Geometry check sheet. Reference: the model listing, model coordinates, mm. A direction names the side the tool comes from. Round coordinates to 2 decimals unless told otherwise and drop trailing zeros. Order: outer loops, then holes, each group sorted by start corner. A loop starts at its lowest first (then second) coordinate and runs counter-clockwise, first axis right, second up.
(1) Cross-section at B-B on z = 23. Enter the section's corners in (x, y).
(2) Cross-section at A-A on x = 0. Enter the section's corners in (y, z), and give its area (3 significant figures).
(3) Draft check along Y on faces 4 (the face through (-17.62, 0.55, 74.7)), 5 (the face through (-0.521, -35.716, 12.325)), 6 (the face through (17.55, 43.02, 36.1)), 7 (the face through (0, -44.45, 35)). Enter one of: pulls with the +Y half, pulls with the -Y half, needs draft (parallel to the pull), parting line crosses it, or undercut.
(4) Thickness scan on L1, parallel to Y at x = 0, z = 9; L2, parallel to X at y = -31.75, z = 5; L3, parallel to Z at x = -0.5, y = 19.05. Record the ranges inside material, lowest first.
(5) Set-up check for faces 1 (the face through (-5.95, 19, 51)), 2 (the face through (0, 44.45, 35)), 3 (the face through (-0.521, 27.784, 12.325)): record each of +Z, -Z, +X, -X, +Y, -Y from which the full face is reachable in a straight line by a thin tool's end or side.
(6) Cross-section at C-C on z = 50.8. Enter the section's corners in (x, y), and give its area (3 significant figures).
(7) Gauge pin test, flat ends, axial feed: P1, Ø9, axis at x = 0, y = 31.75, coming from the -Z side; P2, Ø4, axis at x = 1, y = 30.5, coming from the -Z side; P3, Ø2.5, axis at y = -18, z = 51.5, coming from the +X side. Record the tip position at first contact, or that the pin passes through.
(8) Cross-section at D-D on y = 19.05. Enter the section's corners in (x, z).
from build123d import *

# Parameters (mm, degrees)
F0_W     = 38.1
F0_H     = 88.9
F1_DEPTH = 76.2
F2_R     = 4
F3_DEPTH = 25
F4_R     = 4
F5_DEPTH = 25
F6_R     = 5


with BuildPart() as f1:
    # F0 (on Top) → F1 (new body)
    with BuildSketch(Plane.XY):
        Rectangle(F0_W, F0_H)
    extrude(amount=F1_DEPTH)

    # F2 (on face) → F3 (cut)
    with BuildSketch(Plane(origin=(0, 0, 0), x_dir=(1, 0, 0), z_dir=(0, 0, -1))):
        with Locations((0, 31.75)):
            Circle(F2_R)
        with Locations((0, -31.75)):
            Circle(F2_R)
    extrude(amount=-F3_DEPTH, mode=Mode.SUBTRACT)

    # F4 (on face) → F5 (cut)
    with BuildSketch(Plane.YZ.offset(19.05)):
        with Locations((-19.05, 50.8)):
            Circle(F4_R)
        with Locations((19.05, 50.8)):
            Circle(F4_R)
    extrude(amount=-F5_DEPTH, mode=Mode.SUBTRACT)

    # F6
    f6_edges = [f1.edges().sort_by_distance(p)[0] for p in [
        (-19.05, -44.45, 38.1),
        (19.05, -44.45, 38.1),
        (0, -44.45, 76.2),
        (-19.05, 0, 76.2),
        (19.05, 0, 76.2),
        (19.05, 44.45, 38.1),
        (0, 44.45, 76.2),
        (-19.05, 44.45, 38.1),
    ]]
    fillet(f6_edges, radius=F6_R)


solid = f1.part
Found:
1. outline: (-19.05, -39.45) arc R5 ccw to (-14.05, -44.45) - (14.05, -44.45) arc R5 ccw to (19.05, -39.45) - (19.05, 39.45) arc R5 ccw to (14.05, 44.45) - (-14.05, 44.45) arc R5 ccw to (-19.05, 39.45) - close; hole circle Ø8 at (0, -31.75); hole circle Ø8 at (0, 31.75)
2. outline: (-44.45, 0) - (-35.75, 0) - (-35.75, 25) - (-27.75, 25) - (-27.75, 0) - (27.75, 0) - (27.75, 25) - (35.75, 25) - (35.75, 0) - (44.45, 0) - (44.45, 71.2) arc R5 ccw to (39.45, 76.2) - (-39.45, 76.2) arc R5 ccw to (-44.45, 71.2) - close; hole circle Ø8 at (-19.05, 50.8); hole circle Ø8 at (19.05, 50.8)
2. area: 6,260 mm2
3. face 4: needs draft
3. face 5: undercut
3. face 6: pulls with the +Y half
3. face 7: pulls with the -Y half
4. L1: y = -44.45 to -35.75, -27.75 to 27.75, 35.75 to 44.45
4. L2: x = -19.05 to -4, 4 to 19.05
4. L3: z = 0 to 46.8, 54.8 to 76.2
5. face 1: +X
5. face 2: +Z, -Z, +X, -X, +Y
5. face 3: -Z
6. outline: (-19.05, -39.45) arc R5 ccw to (-14.05, -44.45) - (14.05, -44.45) arc R5 ccw to (19.05, -39.45) - (19.05, -23.05) - (-5.95, -23.05) - (-5.95, -15.05) - (19.05, -15.05) - (19.05, 15.05) - (-5.95, 15.05) - (-5.95, 23.05) - (19.05, 23.05) - (19.05, 39.45) arc R5 ccw to (14.05, 44.45) - (-14.05, 44.45) arc R5 ccw to (-19.05, 39.45) - close
6. area: 2,970 mm2
7. P1: stops at z = 0
7. P2: stops at z = 25
7. P3: stops at x = -5.95
8. outline: (-19.05, 0) - (19.05, 0) - (19.05, 46.8) - (-5.95, 46.8) - (-5.95, 54.8) - (19.05, 54.8) - (19.05, 71.2) arc R5 ccw to (14.05, 76.2) - (-14.05, 76.2) arc R5 ccw to (-19.05, 71.2) - close
